Check sheet for the modelled part. Datum: model origin and axes. Units: mm. A direction names the side the tool comes from. Coordinates: 2 decimals unless noted, no trailing zeros. Loops run counter-clockwise (first coordinate to the right, second up) from the corner with the lowest first, then second, coordinate; pieces in that order, holes last. Notation, with made-up numbers: M -11.75,31 L -7.75,31 A21 cw -7.75,55 Z; hole C 81.25,86 d10. An arc over 180 degrees is marked long. Answer as CSV lines item,"result". Start each with the question number.
from build123d import *

# Parameters (mm, degrees)
EXTRUDE_1_DEPTH     = 10
FILLET_1_R          = 1
SKETCH_3_R          = 1.5
CUT_EXTRUDE_2_DEPTH = 6
SKETCH_2_R          = 1.5
CUT_EXTRUDE_3_DEPTH = 48.916594203


with BuildPart() as part:
    # 草图1 → 凸台-拉伸1 (new body)
    with BuildSketch(Plane.XY):
        with BuildLine():
            Line((-17.046320844, 30), (-12.046320844, 30))
            Line((-12.046320844, 30), (-12.046320844, 1))
            ThreePointArc((-12.046320844, 1), (-11.753427625, 0.292893219), (-11.046320844, 0))
            Line((-11.046320844, 0), (12.953679156, 0))
            ThreePointArc((12.953679156, 0), (13.660785937, 0.292893219), (13.953679156, 1))
            Line((13.953679156, 1), (13.953679156, 30))
            Line((13.953679156, 30), (18.953679156, 30))
            Line((18.953679156, 30), (18.953679156, -4))
            ThreePointArc((18.953679156, -4), (18.660785937, -4.707106781), (17.953679156, -5))
            Line((17.953679156, -5), (-16.046320844, -5))
            ThreePointArc((-16.046320844, -5), (-16.753427625, -4.707106781), (-17.046320844, -4))
            Line((-17.046320844, -4), (-17.046320844, 30))
        make_face()
    extrude(amount=EXTRUDE_1_DEPTH)

    # 圆角1
    fillet_1_edges = [part.edges().sort_by_distance(p)[0] for p in [
        (18.953679156, 30, 5),
        (13.953679156, 30, 5),
        (-12.046320844, 30, 5),
        (-17.046320844, 30, 5),
    ]]
    fillet(fillet_1_edges, radius=FILLET_1_R)

    # 草图3 → 切除-拉伸2 (cut)
    with BuildSketch(Plane.XZ.offset(5)):
        with Locations((0.476839578, 5)):
            Circle(SKETCH_3_R)
    extrude(amount=-CUT_EXTRUDE_2_DEPTH, mode=Mode.SUBTRACT)

    # 草图2 → 切除-拉伸3 (cut, through all)
    with BuildSketch(Plane.ZY.offset(17.046320844)):
        with Locations((5, 12.5)):
            Circle(SKETCH_2_R)
        with Locations((5, 6.5)):
            Circle(SKETCH_2_R)
        with Locations((5, 18.5)):
            Circle(SKETCH_2_R)
    extrude(amount=-CUT_EXTRUDE_3_DEPTH, mode=Mode.SUBTRACT)


solid = part.part
Item 1: Sectioned sample at D-D, the plane z = 7. Record the boundary of the cut face in (x, y).
Item 2: Set-up check for faces 1 (the face through (-12.046, 15, 5)), 2 (the face through (16.419, 5.925, 6.386)): record each of +Z, -Z, +X, -X, +Y, -Y from which the full face is reachable in a straight line by a thin tool's end or side.
Item 3: Sectioned sample at C-C, the plane x = -14.5. Record the boundary of the cut face in (y, z), and give its area (3 significant figures).
Item 4: Sectioned sample at B-B, the plane y = 23. Record the boundary of the cut face in (x, z), and give its area (3 significant figures).
Item 5: Release check for a two-part mould opening along X. For faces 3 (the face through (16, 30, 5)), 4 (the face through (-16.75, 29.71, 5.07)), 5 (the face through (1, 0, 3)) record: released by +X, released by -X, zero draft, split by the parting line, or undercut.
Item 6: Sectioned sample at A-A, the plane y = 12.5. Record the boundary of the cut face in (x, z).
Item 7: Go/stop test with flat-tipped pins: pin 1 (3.5 mm diameter, centred on y = 18.5, z = 5, fed in from +X); pin 2 (3.5 mm diameter, centred on x = 0.48, z = 5, fed in from +Y); pin 3 (1.8 mm diameter, centred on y = 12.5, z = 5, fed in from -X). Record where each tip stops, or that it passes through.
Item 8: Material ranges on line 1 (Y direction, x = -14.2, z = 5); line 2 (X direction, y = 21.5, z = 4.75); line 3 (Y direction, x = -3.5, z = 4.25), recorded low to high. Write a range as from..to.
Reply:
1,outline,"M -17.05,-4 A1 ccw -16.05,-5 L 17.95,-5 A1 ccw 18.95,-4 L 18.95,29 A1 ccw 17.95,30 L 14.95,30 A1 ccw 13.95,29 L 13.95,1 A1 cw 12.95,0 L -11.05,0 A1 cw -12.05,1 L -12.05,29 A1 ccw -13.05,30 L -16.05,30 A1 ccw -17.05,29 Z"
2,face 1,"+Z, -Z, +Y"
2,face 2,"+X, -X"
3,outline,"M -5,0 L 30,0 L 30,10 L -5,10 Z; hole C 6.5,5 d3; hole C 12.5,5 d3; hole C 18.5,5 d3"
3,area,"329 mm²"
4,outline,"M -17.05,0 L -12.05,0 L -12.05,10 L -17.05,10 Z; M 13.95,0 L 18.95,0 L 18.95,10 L 13.95,10 Z"
4,area,"100 mm²"
5,face 3,"zero draft"
5,face 4,"released by -X"
5,face 5,"undercut"
6,outline,"M -17.05,0 L -12.05,0 L -12.05,3.5 L -17.05,3.5 Z; M -17.05,6.5 L -12.05,6.5 L -12.05,10 L -17.05,10 Z; M 13.95,0 L 18.95,0 L 18.95,3.5 L 13.95,3.5 Z; M 13.95,6.5 L 18.95,6.5 L 18.95,10 L 13.95,10 Z"
7,pin 1,"x = 18.95"
7,pin 2,"y = 0"
7,pin 3,"through"
8,line 1,"-5..5, 8..11, 14..17, 20..30"
8,line 2,"-17.05..-12.05, 13.95..18.95"
8,line 3,"-5..0"
